Part print with two shaded views. Sizes in mm from the minimum x, y, z corner. A direction names the side the tool comes from. Round coordinates to 2 decimals unless told otherwise and drop trailing zeros. Write each loop counter-clockwise with the first axis right and the second up, starting at its lowest first coordinate (ties: lowest second). Pieces come first, ordered by that corner, then holes. Notation, with made-up numbers: (77.5, 14.25) - (95.5, 14.25) arc R16 ccw to (95.5, 20.25) - close; hole circle Ø2 at (18, 70.25). An arc over 180 degrees is marked (long way). Answer as a JSON object with one key per item and string values. Group by question number.
Item 1: Two-plate mould, pull along Y, no slides. Class the marked faces 1, 2, 3 and 4: +Y half, -Y half, draft (parallel to the pull), parting line (faces both ways), or undercut.
Item 2: Which spindle directions (+Z, -Z, +X, -X, +Y, -Y) get a long thin tool onto all of the face, cutting with end or side? Do the marked faces 5, 6, 7 and 8. Say none if no direction does.
Item 3: Flat gauge pin, fed straight in: pin 1 (1 mm diameter, centred on y = 6, z = 4, fed in from -X). Where does the tip first touch, or does it go through?
Item 4: Probe line 1 (X direction, y = 3.5, z = 1.4); line 2 (X direction, y = 4.5, z = 3.85); line 3 (Y direction, x = 1.75, z = 5.05). List the from-to ranges inside material, lowest first. Write a range as from..to.
Item 5: Slice it at B-B, the plane z = 4.95. List the corners of the cut face in (x, y) (1 decimal).
Item 6: Slice it at A-A, the plane z = 2.35. List the corners of the cut face in (x, y) (1 decimal).
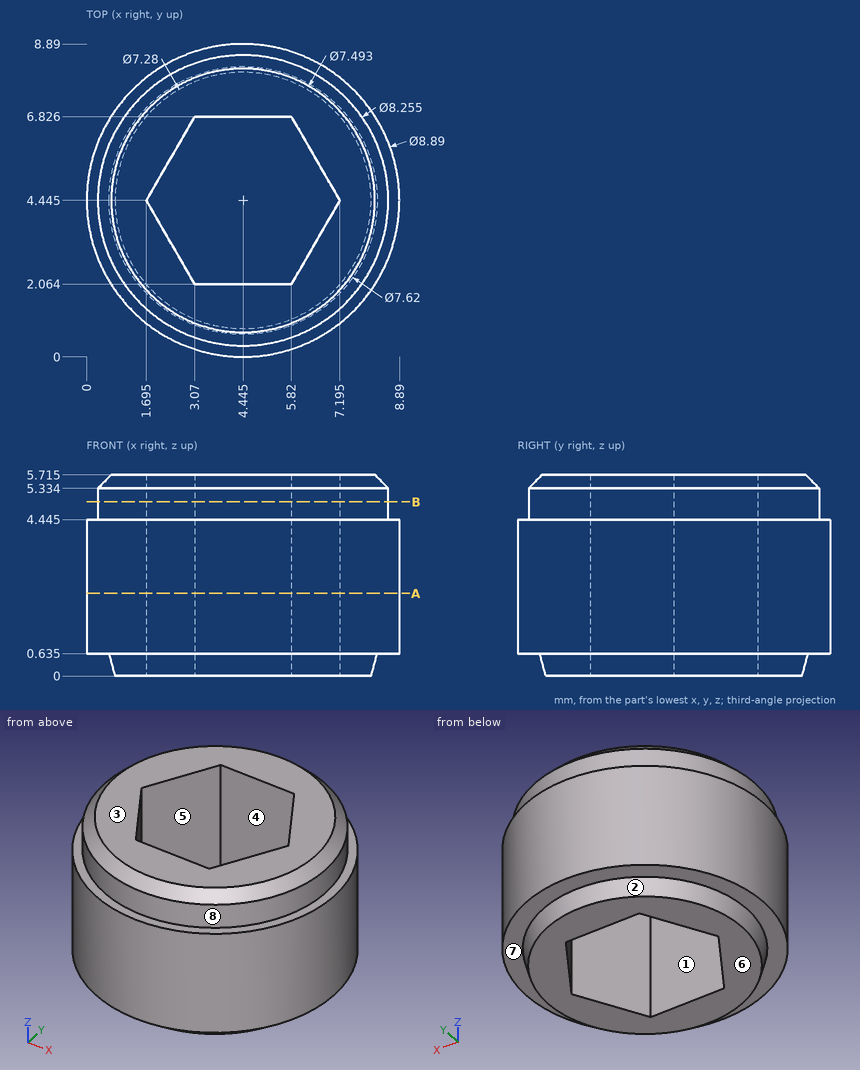
Geometry says:
{
 "1": {"face 1": "undercut", "face 2": "parting line", "face 3": "draft", "face 4": "undercut"},
 "2": {"face 5": "+Z, -Z", "face 6": "-Z, +X, -X, +Y, -Y", "face 7": "-Z", "face 8": "+Z"},
 "3": {"pin 1": "stops at x = 0.13"},
 "4": {"line 1": "x = 0.1..2.24, 6.65..8.79", "line 2": "x = 0..1.73, 7.16..8.89", "line 3": "y = 1.32..4.35, 4.54..7.57"},
 "5": {"outline": "circle Ø8.3 at (4.4, 4.4); hole (1.7, 4.4) - (3.1, 2.1) - (5.8, 2.1) - (7.2, 4.4) - (5.8, 6.8) - (3.1, 6.8) - close"},
 "6": {"outline": "circle Ø8.9 at (4.4, 4.4); hole (1.7, 4.4) - (3.1, 2.1) - (5.8, 2.1) - (7.2, 4.4) - (5.8, 6.8) - (3.1, 6.8) - close"}
}
